Design review of the part built by this model. Coordinates are the model's own, in mm. Face numbers are marked on the shaded views. A direction names the side the tool comes from. Give positions to 0.01 mm unless a question says otherwise; leave off trailing zeros. Write each loop counter-clockwise with the first axis right and the second up, starting at its lowest first coordinate (ties: lowest second). Pieces come first, ordered by that corner, then holes. Notation, with made-up numbers: (36.25, 50) - (59.25, 50) arc R25 ccw to (59.25, 82) - close; hole circle Ø4 at (12, -16). An arc over 180 degrees is marked (long way). Write each question's results on one line, items separated by ' | '. Start each with the question number.
from build123d import *

# Parameters (mm, degrees)
SKETCH1_W               = 850
SKETCH1_H               = 200
BOSS_EXTRUDE1_DEPTH     = 100
SKETCH2_W               = 150
SKETCH2_H               = 200
BOSS_EXTRUDE2_DEPTH     = 200
SKETCH4_W               = 100
SKETCH4_H               = 200
BOSS_EXTRUDE3_DEPTH     = 60
CUT_EXTRUDE1_DEPTH      = 924.309265631
CUT_EXTRUDE1_DEPTH_BACK = 924.309265631
SKETCH3_R               = 38.1
SKETCH3_R_2             = 11.11
SKETCH3_R_3             = 4


with BuildPart() as part:
    # Sketch1 → Boss-Extrude1 (new body)
    with BuildSketch(Plane(origin=(0, 0, 0), x_dir=(1, 0, 0), z_dir=(0, 1, 0))):
        with Locations((425, 100)):
            Rectangle(SKETCH1_W, SKETCH1_H)
    extrude(amount=BOSS_EXTRUDE1_DEPTH)

    # Sketch2 → Boss-Extrude2 (add)
    with BuildSketch(Plane(origin=(0, 100, 0), x_dir=(1, 0, 0), z_dir=(0, 1, 0))):
        with Locations((75, 100)):
            Rectangle(SKETCH2_W, SKETCH2_H)
    extrude(amount=BOSS_EXTRUDE2_DEPTH)

    # Sketch4 → Boss-Extrude3 (add)
    with BuildSketch(Plane(origin=(0, 100, 0), x_dir=(1, 0, 0), z_dir=(0, 1, 0))):
        with Locations((800, 100)):
            Rectangle(SKETCH4_W, SKETCH4_H)
    extrude(amount=BOSS_EXTRUDE3_DEPTH)

    # Sketch3 → Cut-Extrude1 (cut, two sides: drawn at the far end of the back side and taken through both)
    with BuildSketch(Plane.ZY.offset(-CUT_EXTRUDE1_DEPTH_BACK)):
        with Locations((-100, 240)):
            Circle(SKETCH3_R)
        with Locations((-145, 120)):
            Circle(SKETCH3_R_2)
        with Locations(Location((-55, 120, 0), (0, 0, 180))):
            Circle(SKETCH3_R_2)
        with Locations((-100, 140)):
            Circle(SKETCH3_R_3)
    extrude(amount=CUT_EXTRUDE1_DEPTH + CUT_EXTRUDE1_DEPTH_BACK, mode=Mode.SUBTRACT)


solid = part.part
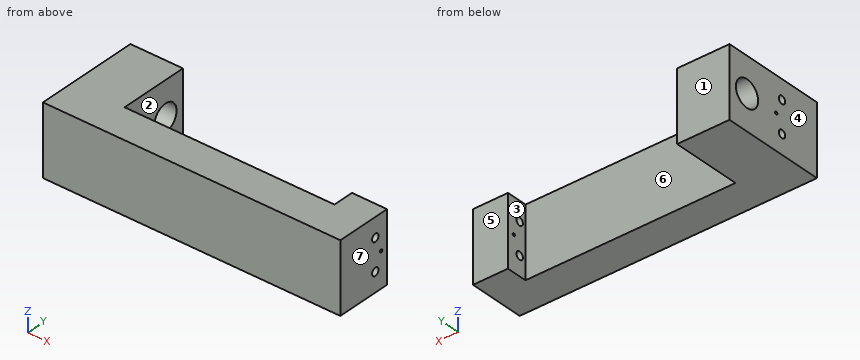
Q1. Add section C-C on y = 259. State the section outline as (x, z) points.
Q2. The part is to be moulded in two halves that separate along X. For the marked faces 1, 2, 3 and 4, say which applies: +X half, -X half, draft (parallel to the pull), parting line (faces both ways), or undercut.
Q3. Add section D-D on x = 406.5. State the section outline as (y, z) points, plus the area to 3 significant figures.
Q4. Add section B-B on x = 766. State the section outline as (y, z) points, plus the area to 3 significant figures.
Q5. For line 1 along Y through (x, z) = (104, -145); line 2 along Z through (x, y) = (112.5, 240); line 3 along Y through (x, z) = (822, -145), list the stretches that pass through material, from the lowest coordinate up. Write a range as [from, to].
Q6. Machinability: for the marked faces 5, 6 and 7, which of the approach directions +Z, -Z, +X, -X, +Y, -Y give a long, thin tool a straight path to every point of the face, cutting with its end or side? Answer none if there is none.
Q7. Insertion check: P1, Ø20, axis at y = 120, z = -55, coming from the -X side; P2, Ø10, axis at y = 221.5, z = -169, coming from the +X side; P3, Ø3, axis at x = 155.5, z = -177.5, coming from the +Y side. Each pin has a flat end and moves straight along its axis. Give the tip position at first contact, or say it passes through.
Q8. Add section A-A on y = 120. State the section outline as (x, z) points.
Result:
1) outline: (0, -200) - (150, -200) - (150, -133.02) - (0, -133.02) - close; (0, -66.98) - (150, -66.98) - (150, 0) - (0, 0) - close
2) face 1: draft | face 2: undercut | face 3: undercut | face 4: -X half
3) outline: (0, -200) - (100, -200) - (100, 0) - (0, 0) - close | area: 20,000 mm²
4) outline: (0, -200) - (160, -200) - (160, 0) - (0, 0) - close; hole circle Ø22.22 at (120, -145); hole circle Ø22.22 at (120, -55); hole circle Ø8 at (140, -100) | area: 31,200 mm²
5) line 1: y = [0, 108.89], [131.11, 300] | line 2: z = [-200, -138.1], [-61.9, 0] | line 3: y = [0, 108.89], [131.11, 160]
6) face 5: +Z, -Z, +X, +Y | face 6: +Z, -Z, +Y | face 7: +Z, -Z, +X, +Y, -Y
7) P1: passes through | P2: stops at x = 150 | P3: stops at y = 100
8) outline: (0, -200) - (150, -200) - (150, -156.11) - (0, -156.11) - close; (0, -133.89) - (150, -133.89) - (150, -66.11) - (0, -66.11) - close; (0, -43.89) - (150, -43.89) - (150, 0) - (0, 0) - close; (750, -200) - (850, -200) - (850, -156.11) - (750, -156.11) - close; (750, -133.89) - (850, -133.89) - (850, -66.11) - (750, -66.11) - close; (750, -43.89) - (850, -43.89) - (850, 0) - (750, 0) - close
